The listing builds one solid part. Answer for the finished solid, in the listing's coordinates (mm). Face numbers are marked on the shaded views. Give positions to 0.01 mm unless a question says otherwise; leave off trailing zeros. Loops run counter-clockwise (first coordinate to the right, second up) from the corner with the lowest first, then second, coordinate; pieces in that order, holes last. Notation, with made-up numbers: (47, 44.5) - (81, 44.5) arc R10 cw to (81, 57.5) - close; hole circle Ø2 at (29, 28). An arc over 180 degrees is marked (long way). One line per item, written item: value. Start each with the question number.
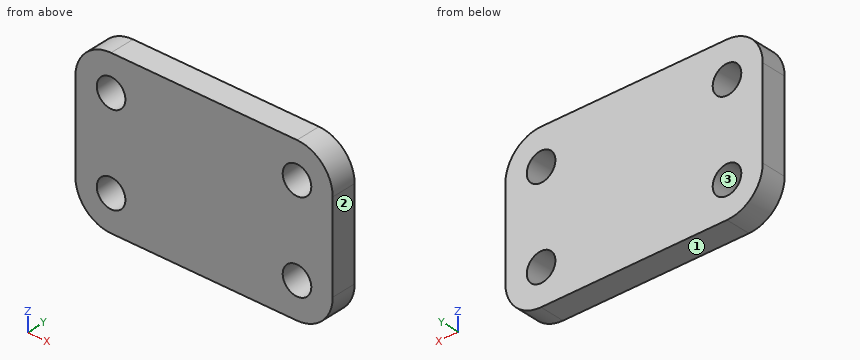
from build123d import *

# Parameters (mm, degrees)
CROQUIS1_W              = 72
CROQUIS1_H              = 45
SALIENTE_EXTRUIR1_DEPTH = 7
REDONDEO1_R             = 10
REDONDEO2_R             = 10
CROQUIS2_R              = 4
CORTAR_EXTRUIR1_DEPTH   = 7


with BuildPart() as part:
    # Croquis1 → Saliente-Extruir1 (new body)
    with BuildSketch(Plane(origin=(0, 0, 0), x_dir=(1, 0, 0), z_dir=(0, 1, 0))):
        Rectangle(CROQUIS1_W, CROQUIS1_H)
    extrude(amount=SALIENTE_EXTRUIR1_DEPTH)

    # Redondeo1
    redondeo1_edges = [part.edges().sort_by_distance(p)[0] for p in [
        (36, 3.5, 22.5),
    ]]
    fillet(redondeo1_edges, radius=REDONDEO1_R)

    # Redondeo2
    redondeo2_edges = [part.edges().sort_by_distance(p)[0] for p in [
        (-36, 3.5, 22.5),
        (-36, 3.5, -22.5),
        (36, 3.5, -22.5),
    ]]
    fillet(redondeo2_edges, radius=REDONDEO2_R)

    # Croquis2 → Cortar-Extruir1 (cut)
    with BuildSketch(Plane(origin=(0, 7, 0), x_dir=(1, 0, 0), z_dir=(0, 1, 0))):
        with Locations(Location((-26, 12.5, 0), (0, 0, 270))):
            Circle(CROQUIS2_R)
        with Locations(Location((-26, -12.5, 0), (0, 0, 270))):
            Circle(CROQUIS2_R)
        with Locations(Location((26, -12.5, 0), (0, 0, 270))):
            Circle(CROQUIS2_R)
        with Locations(Location((26, 12.5, 0), (0, 0, 270))):
            Circle(CROQUIS2_R)
    extrude(amount=-CORTAR_EXTRUIR1_DEPTH, mode=Mode.SUBTRACT)


solid = part.part
1. A cutting plane is placed at A-A (y = 2.75). Determine the outline of the cut face in (x, z), plus the area to 3 significant figures.
2. A flat-ended cylindrical pin translates along its axis: pin 1 (10.5 mm diameter, centred on x = 26, z = -12.5, fed in from +Y). Find the tip coordinate at first contact, or state that the pin passes through.
3. Determine the mould class of the marked faces 1, 2 and 3 for opening direction X: released by +X, released by -X, zero draft, split by the parting line, or undercut.
4. A cutting plane is placed at B-B (z = 18). Determine the outline of the cut face in (x, y).
5. Find the intervals of material crossed by L1, parallel to X at y = 2, z = -12.5; L2, parallel to X at y = 4.75, z = 10; L3, parallel to Z at x = 28.5, y = 6, in increasing order. Write a range as [from, to].
Results below:
1. outline: (-36, -12.5) arc R10 ccw to (-26, -22.5) - (26, -22.5) arc R10 ccw to (36, -12.5) - (36, 12.5) arc R10 ccw to (26, 22.5) - (-26, 22.5) arc R10 ccw to (-36, 12.5) - close; hole circle Ø8 at (-26, -12.5); hole circle Ø8 at (-26, 12.5); hole circle Ø8 at (26, -12.5); hole circle Ø8 at (26, 12.5)
1. area: 2,950 mm^2
2. pin 1: stops at y = 7
3. face 1: zero draft
3. face 2: released by +X
3. face 3: undercut
4. outline: (-34.35, 0) - (34.35, 0) - (34.35, 7) - (-34.35, 7) - close
5. L1: x = [-36, -30], [-22, 22], [30, 36]
5. L2: x = [-36, -29.12], [-22.88, 22.88], [29.12, 36]
5. L3: z = [-22.18, -15.62], [-9.38, 9.38], [15.62, 22.18]
